Geometry: final body of the model. Coordinates: model frame, mm. Coordinates: 2 decimals unless noted, no trailing zeros. Order: outer loops, then holes, each group sorted by start corner. A loop starts at its lowest first (then second) coordinate and runs counter-clockwise, first axis right, second up. Notation, with made-up numbers: (62.5, 57) -> (76.5, 57) arc R25 ccw to (76.5, 92) -> close; hole circle Ø2 at (-25.5, 30). An arc over 180 degrees is marked (long way). Answer in a Markdown table with one row per item. Add a question column.
1) Section query A-A on y = 4. Return the cut outline in (x, z).
2) Section query B-B on z = 2.6. Count the separate pieces of the cut face and the enclosed holes in it, then the cut area to 3 significant figures.
3) Ray query, line 1 (Y direction, x = 2.8, z = 2.5); line 2 (X direction, y = 15, z = 3); line 3 (X direction, y = -9.5, z = 3.1). Return the intervals inside material, ascending. Write a range as from..to.
4) Contact query for flat-ended pins moving along their axis: P1, Ø3, axis at x = 2, y = -19, coming from the -Z side; P2, Ø0.6, axis at y = 21, z = 1, coming from the -X side; P3, Ø0.6, axis at x = 1.5, z = 1, coming from the -Y side. Output: stop coordinate, or through.
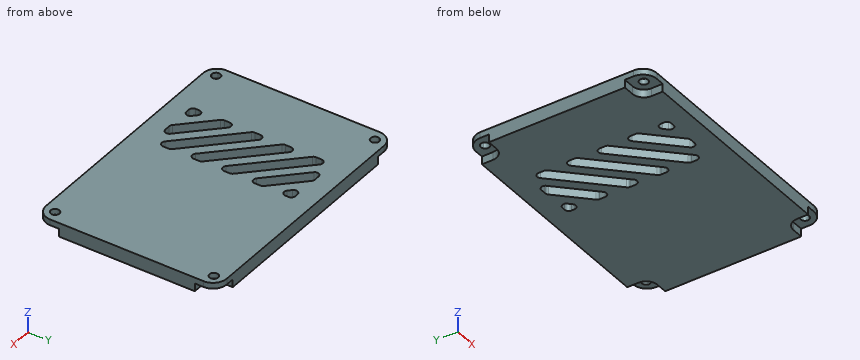
```python
from build123d import *

# Parameters (mm, degrees)
BOSS_EXTRUDE1_DEPTH = 3.5
CUT_EXTRUDE1_DEPTH  = 10
CUT_EXTRUDE2_DEPTH  = 2
CUT_EXTRUDE3_DEPTH  = 4
FILLET2_R           = 1


with BuildPart() as part:
    # Sketch1 → Boss-Extrude1 (new body)
    with BuildSketch(Plane.XY):
        with BuildLine():
            Line((3.5, 23), (61.5, 23))
            ThreePointArc((61.5, 23), (63.974873734, 21.974873734), (65, 19.5))
            Line((65, 19.5), (65, -19.5))
            ThreePointArc((65, -19.5), (63.974873734, -21.974873734), (61.5, -23))
            Line((61.5, -23), (3.5, -23))
            ThreePointArc((3.5, -23), (1.025126266, -21.974873734), (0, -19.5))
            Line((0, -19.5), (0, 19.5))
            ThreePointArc((0, 19.5), (1.025126266, 21.974873734), (3.5, 23))
        make_face()
    extrude(amount=BOSS_EXTRUDE1_DEPTH)

    # Sketch2 → Cut-Extrude1 (cut)
    with BuildSketch(Plane.XY.offset(3.5)):
        with BuildLine():
            ThreePointArc((1.720986059, -20.413843202), (2.022182541, -20.977817459), (2.586156798, -21.279013941))
            ThreePointArc((2.586156798, -21.279013941), (3.577817459, -19.422182541), (1.720986059, -20.413843202))
        make_face()
        with BuildLine():
            ThreePointArc((2.586156798, 21.279013941), (2.022182541, 20.977817459), (1.720986059, 20.413843202))
            ThreePointArc((1.720986059, 20.413843202), (2.236022068, 19.255580129), (3.5, 19.351471863))
            ThreePointArc((3.5, 19.351471863), (3.9, 20.2), (3.5, 21.048528137))
            ThreePointArc((3.5, 21.048528137), (3.069013075, 21.266598315), (2.586156798, 21.279013941))
        make_face()
        with BuildLine():
            ThreePointArc((62.413843202, -21.279013941), (62.977817459, -20.977817459), (63.279013941, -20.413843202))
            ThreePointArc((63.279013941, -20.413843202), (61.422182541, -19.422182541), (62.413843202, -21.279013941))
        make_face()
        with BuildLine():
            ThreePointArc((63.279013941, 20.413843202), (62.977817459, 20.977817459), (62.413843202, 21.279013941))
            ThreePointArc((62.413843202, 21.279013941), (61.422182541, 19.422182541), (63.279013941, 20.413843202))
        make_face()
    extrude(amount=-CUT_EXTRUDE1_DEPTH, mode=Mode.SUBTRACT)

    # Sketch3 → Cut-Extrude2 (cut)
    with BuildSketch(Plane(origin=(0, 0, 0), x_dir=(-1, 0, 0), z_dir=(0, 0, -1))):
        with BuildLine():
            Line((-2.8, -17.3), (0, -17.3))
            Line((0, -17.3), (0, -19.5))
            ThreePointArc((0, -19.5), (-1.025126266, -21.974873734), (-3.5, -23))
            Line((-3.5, -23), (-5.7, -23))
            Line((-5.7, -23), (-5.7, -20.2))
            ThreePointArc((-5.7, -20.2), (-4.850609665, -18.149390335), (-2.8, -17.3))
        make_face()
        with BuildLine():
            Line((-2.8, 17.3), (0, 17.3))
            Line((0, 17.3), (0, 19.5))
            ThreePointArc((0, 19.5), (-1.025126266, 21.974873734), (-3.5, 23))
            Line((-3.5, 23), (-5.7, 23))
            Line((-5.7, 23), (-5.7, 20.2))
            ThreePointArc((-5.7, 20.2), (-4.850609665, 18.149390335), (-2.8, 17.3))
        make_face()
        with BuildLine():
            Line((-59.3, 20.2), (-59.3, 23))
            Line((-59.3, 23), (-61.5, 23))
            ThreePointArc((-61.5, 23), (-63.974873734, 21.974873734), (-65, 19.5))
            Line((-65, 19.5), (-65, 17.3))
            Line((-65, 17.3), (-62.2, 17.3))
            ThreePointArc((-62.2, 17.3), (-60.149390335, 18.149390335), (-59.3, 20.2))
        make_face()
        with BuildLine():
            Line((-62.2, -17.3), (-65, -17.3))
            Line((-65, -17.3), (-65, -19.5))
            ThreePointArc((-65, -19.5), (-63.974873734, -21.974873734), (-61.5, -23))
            Line((-61.5, -23), (-59.3, -23))
            Line((-59.3, -23), (-59.3, -20.2))
            ThreePointArc((-59.3, -20.2), (-60.149390335, -18.149390335), (-62.2, -17.3))
        make_face()
    extrude(amount=-CUT_EXTRUDE2_DEPTH, mode=Mode.SUBTRACT)

    # Sketch4 → Cut-Extrude3 (cut)
    with BuildSketch(Plane(origin=(0, 0, 0), x_dir=(-1, 0, 0), z_dir=(0, 0, -1))):
        Polygon((-25.757359313, 18), (-30, 18), (-30, 13.757359313), align=None)
        Polygon((-17.97918472, 18), (-22.221825407, 18), (-30, 10.221825407), (-30, 5.97918472), align=None)
        Polygon((-15, 17.443650814), (-30, 2.443650814), (-30, -1.798989873), (-15, 13.201010127), align=None)
        Polygon((-15, 9.665476221), (-30, -5.334523779), (-30, -9.577164466), (-15, 5.422835534), align=None)
        Polygon((-15, 1.887301628), (-30, -13.112698372), (-30, -17.355339059), (-15, -2.355339059), align=None)
        Polygon((-15, -10.133513652), (-15, -5.890872965), (-27.109127035, -18), (-22.866486348, -18), align=None)
        Polygon((-15, -18), (-15, -13.669047558), (-19.330952442, -18), align=None)
    extrude(amount=-CUT_EXTRUDE3_DEPTH, mode=Mode.SUBTRACT)

    # Fillet2
    fillet2_edges = [part.edges().sort_by_distance(p)[0] for p in [
        (30, -9.577164466, 1.75),
        (30, -5.334523779, 1.75),
        (15, 9.665476221, 1.75),
        (15, 5.422835534, 1.75),
        (30, -17.355339059, 1.75),
        (30, -13.112698372, 1.75),
        (15, 1.887301628, 1.75),
        (15, -2.355339059, 1.75),
        (30, 5.97918472, 1.75),
        (30, 10.221825407, 1.75),
        (22.221825407, 18, 1.75),
        (17.97918472, 18, 1.75),
        (30, -1.798989873, 1.75),
        (30, 2.443650814, 1.75),
        (15, 17.443650814, 1.75),
        (15, 13.201010127, 1.75),
        (19.330952442, -18, 1.75),
        (15, -13.669047558, 1.75),
        (15, -18, 1.75),
        (22.866486348, -18, 1.75),
        (27.109127035, -18, 1.75),
        (15, -5.890872965, 1.75),
        (15, -10.133513652, 1.75),
        (30, 13.757359313, 1.75),
        (30, 18, 1.75),
        (25.757359313, 18, 1.75),
    ]]
    fillet(fillet2_edges, radius=FILLET2_R)


solid = part.part
```
Result:
| question | item | result |
|---|---|---|
| 1 | outline | (0, 0) -> (16.42, 0) -> (16.42, 3.5) -> (0, 3.5) -> close; (20.67, 0) -> (24.2, 0) -> (24.2, 3.5) -> (20.67, 3.5) -> close; (28.44, 0) -> (65, 0) -> (65, 3.5) -> (28.44, 3.5) -> close |
| 2 | separate pieces | 1 |
| 2 | enclosed holes | 11 |
| 2 | area | 2,690 mm2 |
| 3 | line 1 | -22.93..-21.3, -19.1..19.1, 21.3..22.93 |
| 3 | line 2 | 0..15, 17.44..20.98, 25.22..65 |
| 3 | line 3 | 0..15, 18.61..22.14, 26.39..65 |
| 4 | P1 | z = 2 |
| 4 | P2 | x = 5.7 |
| 4 | P3 | y = -17.3 |
